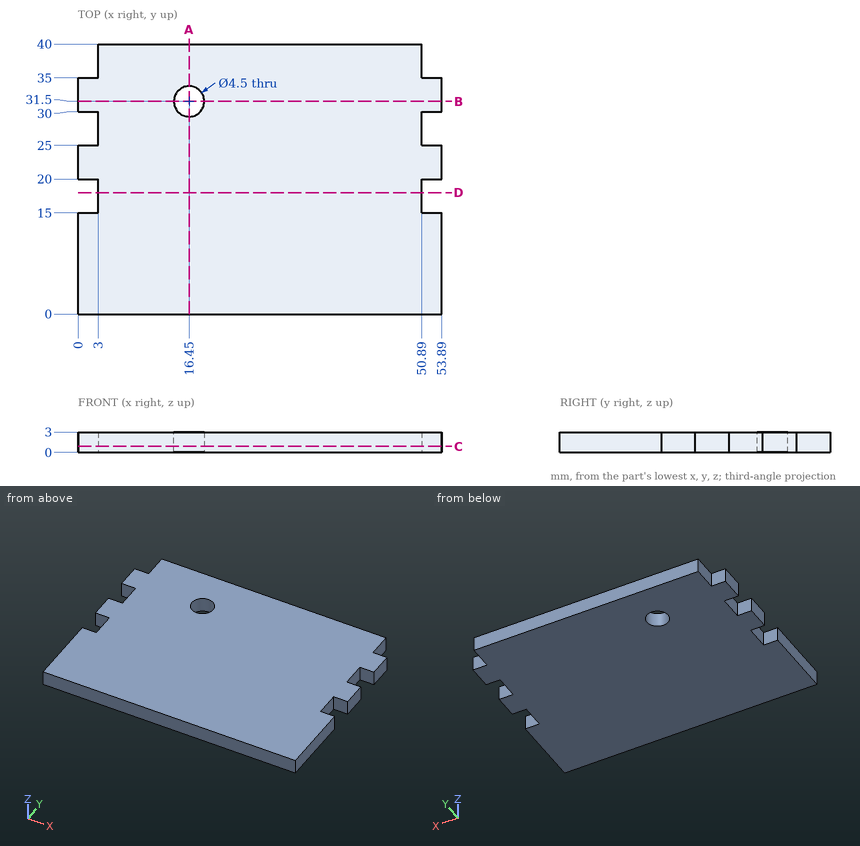
Study the drawing (mm; zero at the part's minimum x, y, z) and answer. Coordinates: 2 decimals unless noted, no trailing zeros. Write each loop counter-clockwise with the first axis right and the second up, starting at its lowest first coordinate (ties: lowest second). Pieces come first, ordered by that corner, then holes.
Q1. Find the intervals of material crossed by line 1 along Y through (x, z) = (16.45, 1.85); line 2 along X through (y, z) = (27, 2.55); line 3 along X through (y, z) = (30.5, 0.15), in increasing order.
Returned:
line 1: y = 0 to 29.25, 33.75 to 40
line 2: x = 3 to 50.89
line 3: x = 0 to 14.43, 18.47 to 53.89
Q2. Section A-A, the plane x = 16.45 is taken. Write down the section's boundary in (y, z).
Returned:
outline: (0, 0) - (29.25, 0) - (29.25, 3) - (0, 3) - close; (33.75, 0) - (40, 0) - (40, 3) - (33.75, 3) - close
Q3. Section B-B, the plane y = 31.5 is taken. Write down the section's boundary in (x, z), then the cut area to 3 significant figures.
Returned:
outline: (0, 0) - (14.2, 0) - (14.2, 3) - (0, 3) - close; (18.7, 0) - (53.89, 0) - (53.89, 3) - (18.7, 3) - close
area: 148 mm2
Q4. Section C-C, the plane z = 0.9 is taken. Write down the section's boundary in (x, y).
Returned:
outline: (0, 0) - (53.89, 0) - (53.89, 15) - (50.89, 15) - (50.89, 20) - (53.89, 20) - (53.89, 25) - (50.89, 25) - (50.89, 30) - (53.89, 30) - (53.89, 35) - (50.89, 35) - (50.89, 40) - (3, 40) - (3, 35) - (0, 35) - (0, 30) - (3, 30) - (3, 25) - (0, 25) - (0, 20) - (3, 20) - (3, 15) - (0, 15) - close; hole circle Ø4.5 at (16.45, 31.5)
Q5. Given P1, Ø1.5, axis at y = 37.5, z = 1.5, coming from the +X side; P2, Ø0.9, axis at x = 52, z = 1, coming from the +Y side; P3, Ø1.5, axis at y = 38.5, z = 1, coming from the -X side, each flat-ended and moving along its own axis, determine where each tip first touches the part or whether it passes through.
Returned:
P1: stops at x = 50.89
P2: stops at y = 35
P3: stops at x = 3
Q6. Section D-D, the plane y = 18 is taken. Write down the section's boundary in (x, z), then the cut area to 3 significant figures.
Returned:
outline: (3, 0) - (50.89, 0) - (50.89, 3) - (3, 3) - close
area: 144 mm2
